For this review, take the finished solid that the model builds, in its own axes (mm). Face numbers are marked on the shaded views. A direction names the side the tool comes from. Coordinates: 2 decimals unless noted, no trailing zeros. Loops run counter-clockwise (first coordinate to the right, second up) from the corner with the lowest first, then second, coordinate; pieces in that order, holes last. Notation, with made-up numbers: M 24.5,47.25 L 66.5,47.25 A5 ccw 66.5,55.25 Z; hole C 44,24 d5. An arc over 180 degrees is marked long. Write each question's results on one line, items separated by ' | '. Start each with the question number.
```python
from build123d import *

# Parameters (mm, degrees)
SKETCH1_W           = 120
SKETCH1_H           = 90
BOSS_EXTRUDE1_DEPTH = 10
BOSS_EXTRUDE2_DEPTH = 4
BOSS_EXTRUDE3_DEPTH = 4


with BuildPart() as part:
    # Sketch1 → Boss-Extrude1 (new body)
    with BuildSketch(Plane(origin=(0, 0, 0), x_dir=(1, 0, 0), z_dir=(0, 1, 0))):
        with Locations((60, 45)):
            Rectangle(SKETCH1_W, SKETCH1_H)
    extrude(amount=BOSS_EXTRUDE1_DEPTH)

    # Sketch2 → Boss-Extrude2 (add)
    with BuildSketch(Plane(origin=(0, 10, 0), x_dir=(1, 0, 0), z_dir=(0, 1, 0))):
        Polygon((10, 70), (20, 80), (80, 80), (115, 45), (80, 10), (20, 10), (10, 20), align=None)
    extrude(amount=BOSS_EXTRUDE2_DEPTH)

    # Sketch3 → Boss-Extrude3 (add)
    with BuildSketch(Plane(origin=(0, 18, 0), x_dir=(-1, 0, 0), z_dir=(0, -1, 0))):
        Polygon((-10, 45), (-34.14221937, 70), (-74.652034735, 70), (-83.534243972, 61.422550244), (-83.534243972, 43.169206873), (-83.534243972, 28.58424312), (-74.645, 20), (-35, 20), align=None)
    extrude(amount=BOSS_EXTRUDE3_DEPTH)


solid = part.part
```
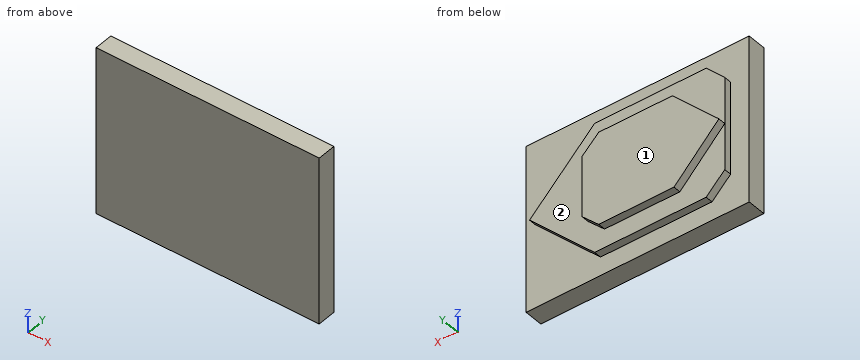
Q1. Take a section at A-A, the plane x = 51.5. Give the boundary of the cut face in (y, z), then the cut area to 3 significant figures.
Q2. To check wall thickness, follow line 1 along Y through (x, z) = (99, -44.5); line 2 along Z through (x, y) = (48, 11); line 3 along Z through (x, y) = (71, 15). State the ranges of each line that lie inside material, in increasing order.
Q3. For the marked faces 1 and 2, list the 3-axis set-ups (+Z, -Z, +X, -X, +Y, -Y) from which the entire face can be reached by the end or side of a thin tool; tool diameter is ignored.
Q4. Take a section at C-C, the plane z = -43.5. Give the boundary of the cut face in (x, y), then the cut area to 3 significant figures.
Q5. Insertion check: P1, Ø3, axis at y = 16, z = -51.5, coming from the +X side; P2, Ø2, axis at x = 54, y = 12.5, coming from the +Z side; P3, Ø1.2, axis at x = 45.5, y = 16.5, coming from the +Z side; P4, Ø1, axis at y = 10, z = -52, coming from the -X side. Each pin has a flat end and moves straight along its axis. Give the tip position at first contact, or say it passes through.
Q6. Take a section at B-B, the plane y = 11.5. Give the boundary of the cut face in (x, z).
Q7. Take a section at D-D, the plane x = 98. Give the boundary of the cut face in (y, z).
Results:
1) outline: M 0,-90 L 10,-90 L 10,-80 L 14,-80 L 14,-70 L 18,-70 L 18,-20 L 14,-20 L 14,-10 L 10,-10 L 10,0 L 0,0 Z | area: 1,380 mm^2
2) line 1: 0 to 14 | line 2: -80 to -10 | line 3: -70 to -20
3) face 1: +Z, -Z, +X, -X, +Y | face 2: +Y
4) outline: M 0,0 L 120,0 L 120,10 L 113.5,10 L 113.5,14 L 83.53,14 L 83.53,18 L 11.5,18 L 11.5,14 L 10,14 L 10,10 L 0,10 Z | area: 1,900 mm^2
5) P1: x = 83.53 | P2: z = -10 | P3: z = -20 | P4: x = 0
6) outline: M 10,-70 L 20,-80 L 80,-80 L 115,-45 L 80,-10 L 20,-10 L 10,-20 Z
7) outline: M 0,-90 L 10,-90 L 10,-62 L 14,-62 L 14,-28 L 10,-28 L 10,0 L 0,0 Z
